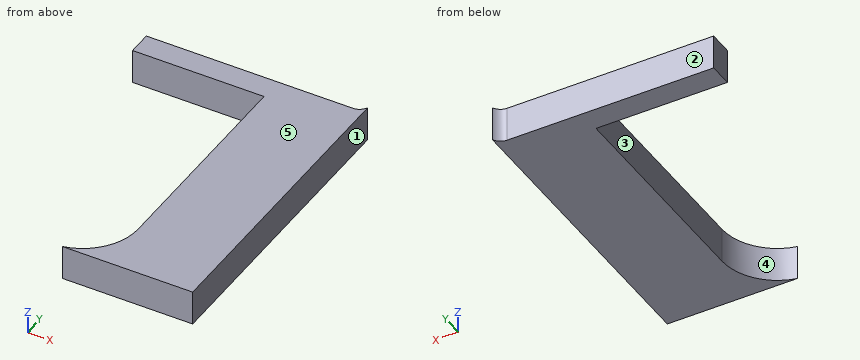
from build123d import *

# Parameters (mm, degrees)
ESTRUSIONE_ESTRUSIONE1_DEPTH = 6.4


with BuildPart() as part:
    # Schizzo1 → Estrusione-Estrusione1 (new body)
    with BuildSketch(Plane.XY):
        with BuildLine():
            Line((29, -3.2), (29, -7.6))
            Line((29, -7.6), (53.2, -7.6))
            Line((53.2, -7.6), (53.2, -47.8))
            ThreePointArc((53.2, -47.8), (50.891189589, -54.262903904), (45.009975124, -57.8))
            Line((45.009975124, -57.8), (69, -57.8))
            Line((69, -57.8), (69, -1.916515139))
            ThreePointArc((69, -1.916515139), (68.188205936, -2.851530894), (67, -3.2))
            Line((67, -3.2), (29, -3.2))
        make_face()
    extrude(amount=ESTRUSIONE_ESTRUSIONE1_DEPTH)


solid = part.part
Read the model definition and answer for the solid it produces. Units are mm, in the model's axes. Face numbers are marked on the shaded views. A direction names the side the tool comes from. Coordinates: 2 decimals unless noted, no trailing zeros. Order: outer loops, then holes, each group sorted by start corner. A loop starts at its lowest first (then second) coordinate and runs counter-clockwise, first axis right, second up. Notation, with made-up numbers: (85, -24) -> (143, -24) arc R18 cw to (143, -10) -> close; hole circle Ø9 at (54, -9.75). An arc over 180 degrees is marked (long way). Answer as a JSON object with one key per item and string values.
1) A cutting plane is placed at A-A, the plane x = 46. Determine the outline of the cut face in (y, z), plus the area to 3 significant figures.
Model answer:
{"outline": "(-57.8, 0) -> (-57.55, 0) -> (-57.55, 6.4) -> (-57.8, 6.4) -> close; (-7.6, 0) -> (-3.2, 0) -> (-3.2, 6.4) -> (-7.6, 6.4) -> close", "area": "29.8 mm²"}
2) A tool of negligible diameter and unlimited length cuts with its end or side. For the marked faces 4 and 5, from which of +Z, -Z, +X, -X, +Y, -Y can it reach the whole face along a straight path? Write none if from no direction.
Model answer:
{"face 4": "+Z, -Z, -X", "face 5": "+Z, +X, -X, +Y, -Y"}
3) Each of these flat-tipped pins is pushed along its axis until it touches: pin 1 (2 mm diameter, centred on y = -12.5, z = 1, fed in from -X); pin 2 (1.5 mm diameter, centred on x = 65, z = 2.5, fed in from +Y). Where does it stop, or does it pass through?
Model answer:
{"pin 1": "stops at x = 53.2", "pin 2": "stops at y = -3.2"}
4) A cutting plane is placed at D-D, the plane x = 64. Determine the outline of the cut face in (y, z), plus the area to 3 significant figures.
Model answer:
{"outline": "(-57.8, 0) -> (-3.2, 0) -> (-3.2, 6.4) -> (-57.8, 6.4) -> close", "area": "349 mm²"}
5) A cutting plane is placed at B-B, the plane z = 2.75. Determine the outline of the cut face in (x, y).
Model answer:
{"outline": "(29, -7.6) -> (53.2, -7.6) -> (53.2, -47.8) arc R10.2 cw to (45.01, -57.8) -> (69, -57.8) -> (69, -1.92) arc R2.2 cw to (67, -3.2) -> (29, -3.2) -> close"}
6) The mould has two halves that part along Y. Classify the marked faces 1, 2 and 3: released by +Y, released by -Y, zero draft, split by the parting line, or undercut.
Model answer:
{"face 1": "zero draft", "face 2": "released by +Y", "face 3": "undercut"}
7) Consider line 1 along Y through (x, z) = (60.5, 2.75); line 2 along Y through (x, z) = (38.5, 2.5); line 3 along X through (y, z) = (-29, 4.5). Determine where each line is inside the solid, lowest interval first. Write a range as from..to.
Model answer:
{"line 1": "y = -57.8..-3.2", "line 2": "y = -7.6..-3.2", "line 3": "x = 53.2..69"}
8) A cutting plane is placed at C-C, the plane y = -28.5. Determine the outline of the cut face in (x, z), plus the area to 3 significant figures.
Model answer:
{"outline": "(53.2, 0) -> (69, 0) -> (69, 6.4) -> (53.2, 6.4) -> close", "area": "101 mm²"}
